Geometry: see drawing. Coordinates: mm, zero at the bounding-box minimum. A direction names the side the tool comes from. Coordinates: 2 decimals unless noted, no trailing zeros. Loops run counter-clockwise (first coordinate to the right, second up) from the corner with the lowest first, then second, coordinate; pieces in that order, holes last. Notation, with made-up numbers: (-35.75, 13.25) -> (-22.75, 13.25) arc R34 ccw to (-22.75, 45.25) -> close; hole circle Ø5 at (4, 35). An arc over 180 degrees is marked (long way). Put each result on its own line as item: value. Start each with the question number.
1) Contact query for flat-ended pins moving along their axis: P1, Ø12, axis at x = 22, z = 78.5, coming from the -Y side; P2, Ø8, axis at x = 29.5, z = 74.5, coming from the -Y side (1 decimal); P3, Ø4, axis at y = 23.5, z = 62, coming from the -X side; P4, Ø7.5, axis at x = 19.5, z = 101.5, coming from the -Y side. Output: stop coordinate, or through.
2) Cut plane A-A (y = 19.05). State how many separate pieces and enclosed holes the cut face has, plus the area to 3 significant figures.
3) Cut plane C-C (x = 19.05). Return the cut outline in (y, z) (1 decimal).
4) Material intervals for L1, parallel to Z at x = 26, y = 24 (1 decimal); L2, parallel to Z at x = 23, y = 21 (1 decimal); L3, parallel to Z at x = 16.5, y = 21.5 (1 decimal), sorted ascending.
5) Cut plane D-D (x = 30). Return the cut outline in (y, z) (1 decimal).
6) Set-up query: the marked faces 1, 2, 3 and 4. Return all of +Z, -Z, +X, -X, +Y, -Y with unobstructed straight access to the full face (end or side cutting, diameter ignored); none if empty.
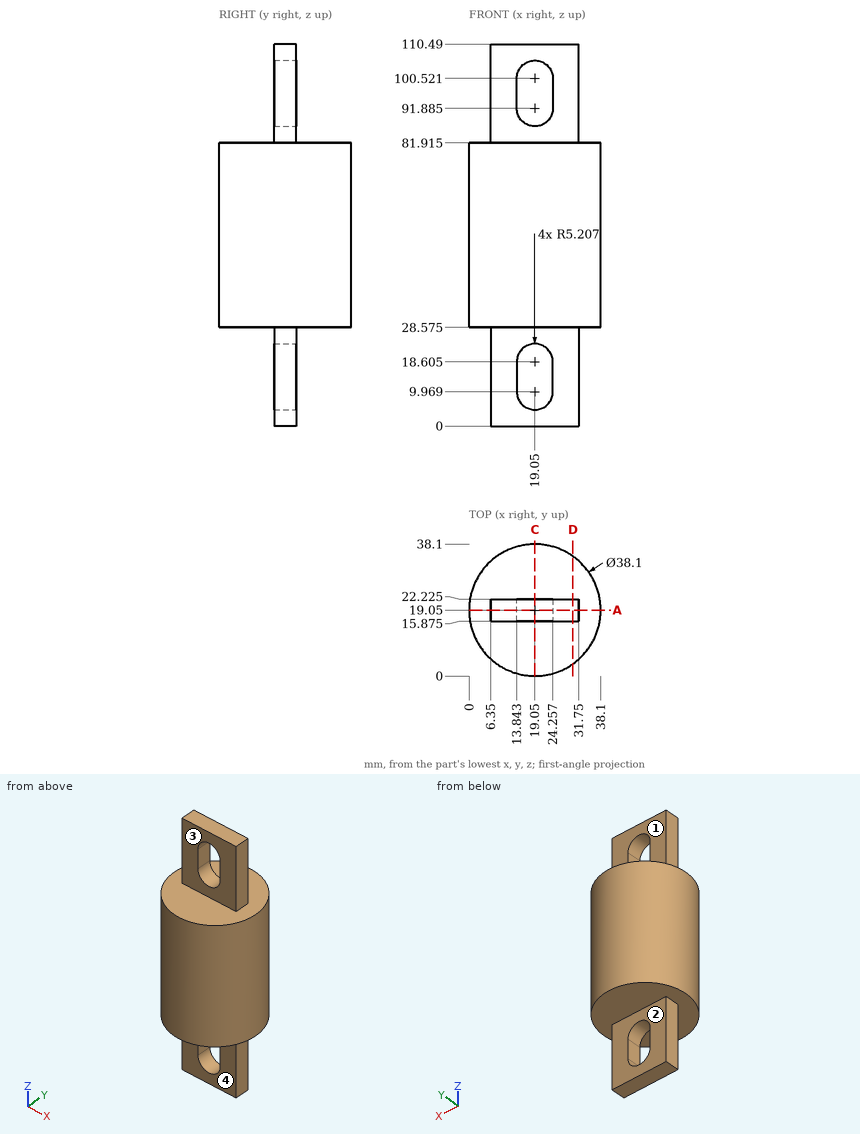
Results found:
1. P1: stops at y = 0
1. P2: stops at y = 1.1
1. P3: stops at x = 0.16
1. P4: passes through
2. separate pieces: 1
2. enclosed holes: 2
2. area: 3,130 mm2
3. outline: (0, 28.6) -> (15.9, 28.6) -> (15.9, 23.8) -> (22.2, 23.8) -> (22.2, 28.6) -> (38.1, 28.6) -> (38.1, 81.9) -> (22.2, 81.9) -> (22.2, 86.7) -> (15.9, 86.7) -> (15.9, 81.9) -> (0, 81.9) -> close; (15.9, 0) -> (22.2, 0) -> (22.2, 4.8) -> (15.9, 4.8) -> close; (15.9, 105.7) -> (22.2, 105.7) -> (22.2, 110.5) -> (15.9, 110.5) -> close
4. L1: z = 28.6 to 81.9
4. L2: z = 0 to 6.6, 22 to 88.5, 103.9 to 110.5
4. L3: z = 0 to 5.4, 23.1 to 87.3, 105.1 to 110.5
5. outline: (3.5, 28.6) -> (15.9, 28.6) -> (15.9, 0) -> (22.2, 0) -> (22.2, 28.6) -> (34.6, 28.6) -> (34.6, 81.9) -> (22.2, 81.9) -> (22.2, 110.5) -> (15.9, 110.5) -> (15.9, 81.9) -> (3.5, 81.9) -> close
6. face 1: +Z, +X, -X, +Y
6. face 2: -Z, +X, -X, +Y
6. face 3: +Z, +X, -X, -Y
6. face 4: -Z, +X, -X, -Y
